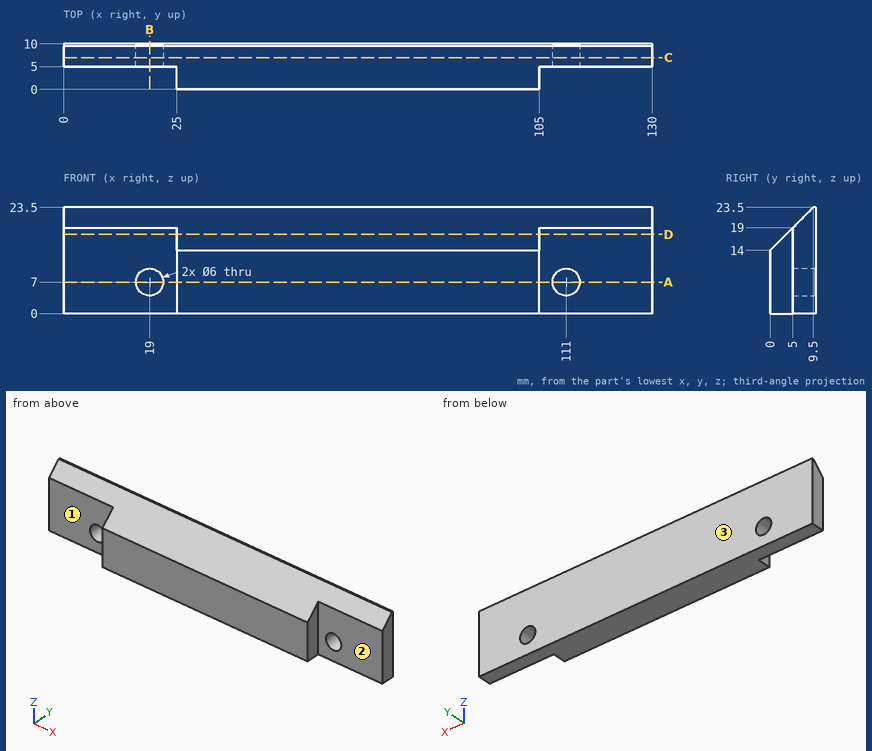
Answer from the drawing. Dimensions are ordinates in mm from the lowest x, y and z of the part. A direction names the side the tool comes from. Round coordinates to 2 decimals unless told otherwise and drop trailing zeros. Order: outer loops, then holes, each group sorted by start corner. A loop starts at its lowest first (then second) coordinate and runs counter-clockwise, first axis right, second up.
1) The part is cut by section D-D on z = 17.5. Write down the section's boundary in (x, y).
2) The part is cut by section A-A on z = 7. Write down the section's boundary in (x, y).
3) The part is cut by section C-C on y = 7. Write down the section's boundary in (x, z).
4) For the marked faces 1, 2 and 3, determine the directions among +Z, -Z, +X, -X, +Y, -Y from which every point of the face is accessible in a straight line to the end or side of a thin tool.
5) Flat-ended cylindrical pins translate along their axes: pin 1 (5 mm diameter, centred on x = 111, z = 7, fed in from +Y); pin 2 (9.5 mm diameter, centred on x = 119.5, z = 6.5, fed in from -Y); pin 3 (5.5 mm diameter, centred on y = 2, z = 6.5, fed in from -X). Find the tip coordinate at first contact, or state that the pin passes through.
6) Straight lines are drawn through the part: L1, parallel to X at y = 6.05, z = 7; L2, parallel to Y at x = 6.5, z = 13.5; L3, parallel to X at y = 1.25, z = 10. For each, find the intervals that lie inside material, in ascending order.
7) The part is cut by section B-B on x = 19. Write down the section's boundary in (y, z).
Resolved:
1. outline: (0, 5) - (25, 5) - (25, 3.5) - (105, 3.5) - (105, 5) - (130, 5) - (130, 10) - (0, 10) - close
2. outline: (0, 5) - (16, 5) - (16, 10) - (0, 10) - close; (22, 5) - (25, 5) - (25, 0) - (105, 0) - (105, 5) - (108, 5) - (108, 10) - (22, 10) - close; (114, 5) - (130, 5) - (130, 10) - (114, 10) - close
3. outline: (0, 0) - (130, 0) - (130, 21) - (0, 21) - close; hole circle Ø6 at (19, 7); hole circle Ø6 at (111, 7)
4. face 1: +Z, -Z, -X, -Y
4. face 2: +Z, -Z, +X, -Y
4. face 3: +Z, -Z, +X, -X, +Y
5. pin 1: passes through
5. pin 2: stops at y = 5
5. pin 3: stops at x = 25
6. L1: x = 0 to 16, 22 to 108, 114 to 130
6. L2: y = 5 to 10
6. L3: x = 25 to 105
7. outline: (5, 0) - (10, 0) - (10, 4) - (5, 4) - close; (5, 10) - (10, 10) - (10, 23.5) - (9.5, 23.5) - (5, 19) - close
